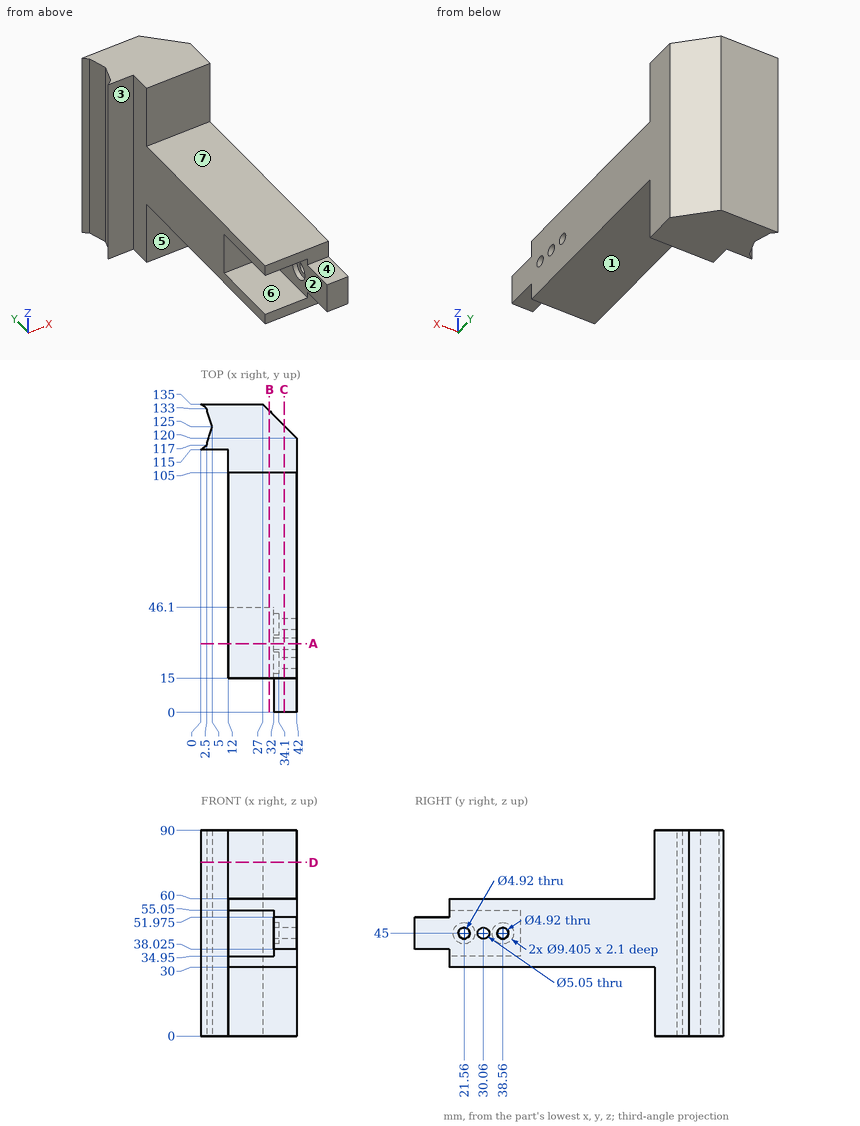
Answer from the drawing. Dimensions are ordinates in mm from the lowest x, y and z of the part. A direction names the side the tool comes from. Coordinates: 2 decimals unless noted, no trailing zeros. Loops run counter-clockwise (first coordinate to the right, second up) from the corner with the lowest first, then second, coordinate; pieces in that order, holes last.
1) Section D-D (z = 76) is taken. Give the vertices of the cut face in (x, y), plus the area to 4 significant figures.
Results:
outline: (0, 115) - (12, 115) - (12, 105) - (42, 105) - (42, 120) - (27, 135) - (0, 135) - (2.5, 133) - (5, 125) - (2.5, 117) - close
area: 962.5 mm2
2) Flat-ended cylindrical pins translate along their axes: pin 1 (11 mm diameter, centred on y = 21.56, z = 45, fed in from -X); pin 2 (15 mm diameter, centred on x = 33, y = 40, fed in from -Z); pin 3 (1 mm diameter, centred on x = 31, z = 16.5, fed in from +Y); pin 4 (22 mm diameter, centred on x = 25.5, z = 43.5, fed in from -Y). Find the tip coordinate at first contact, or state that the pin passes through.
Results:
pin 1: stops at x = 32
pin 2: stops at z = 30
pin 3: stops at y = 131.5
pin 4: stops at y = 0
3) Section C-C (x = 36.5) is taken. Give the vertices of the cut face in (y, z) (3 decimals).
Results:
outline: (0, 38.025) - (15, 38.025) - (15, 30) - (105, 30) - (105, 0) - (125.5, 0) - (125.5, 90) - (105, 90) - (105, 60) - (15, 60) - (15, 51.975) - (0, 51.975) - close; hole circle Ø4.92 at (21.56, 45); hole circle Ø5.05 at (30.06, 45); hole circle Ø4.92 at (38.56, 45)
4) Section B-B (x = 30) is taken. Give the vertices of the cut face in (y, z), plus the area to 3 significant figures.
Results:
outline: (15, 30) - (105, 30) - (105, 0) - (132, 0) - (132, 90) - (105, 90) - (105, 60) - (15, 60) - (15, 55.05) - (46.1, 55.05) - (46.1, 34.95) - (15, 34.95) - close
area: 4,500 mm2
5) For the marked faces 1, 2, 3 and 4, determine the directions among +Z, -Z, +X, -X, +Y, -Y from which every point of the face is accessible in a straight line to the end or side of a thin tool.
Results:
face 1: -Z, +X, -X, -Y
face 2: -X, -Y
face 3: +Z, -Z, -X, -Y
face 4: +Z, +X, -X, -Y
6) Section A-A (y = 30.06) is taken. Give the vertices of the cut face in (x, z) (3 decimals), plus the area to 4 significant figures.
Results:
outline: (12, 30) - (42, 30) - (42, 42.475) - (32, 42.475) - (32, 34.95) - (12, 34.95) - close; (12, 55.05) - (32, 55.05) - (32, 47.525) - (42, 47.525) - (42, 60) - (12, 60) - close
area: 447.5 mm2
7) Consider probe 1 along Z at (x, y) = (28, 41); probe 2 along Y at (x, z) = (39, 45) (3 decimals); probe 3 along Z at (x, y) = (39, 30). Determine where each line is inside the solid, lowest interval first.
Results:
probe 1: z = 30 to 34.95, 55.05 to 60
probe 2: y = 0 to 19.1, 24.02 to 27.535, 32.585 to 36.1, 41.02 to 123
probe 3: z = 30 to 42.48, 47.52 to 60
8) For a pull along Z with two mould halves and no side action, classify the marked faces 5, 6 and 7 as +Z half, -Z half, draft (parallel to the pull), parting line (faces both ways), or undercut.
Results:
face 5: draft
face 6: undercut
face 7: +Z half
